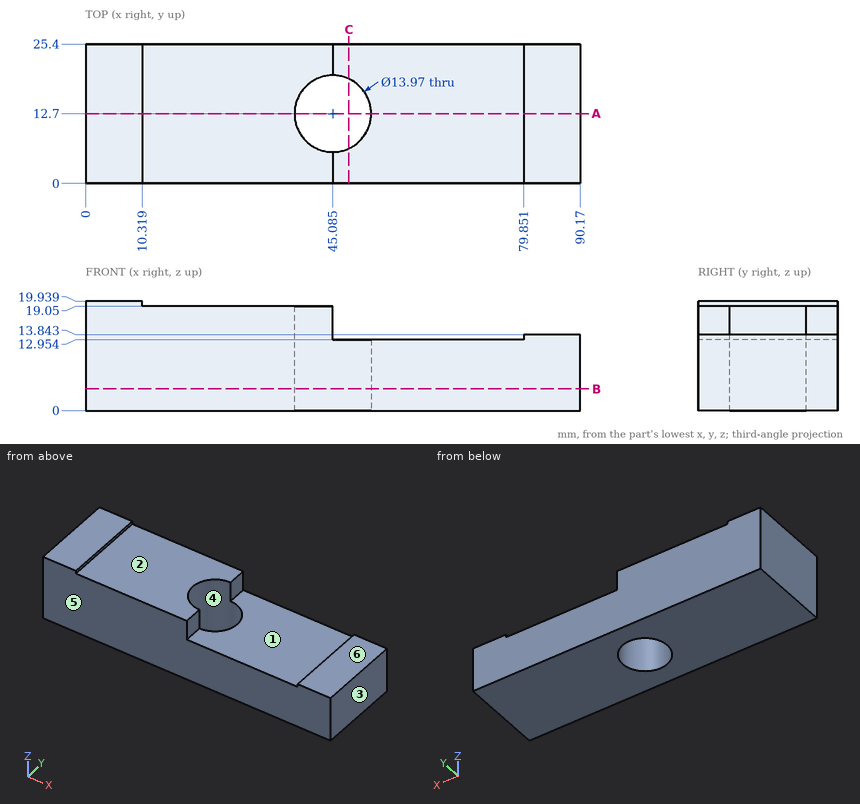
The drawing under review shows one solid part. Ordinate dimensions are in mm from its lowest x, y, z. A direction names the side the tool comes from. Round coordinates to 2 decimals unless told otherwise and drop trailing zeros. Order: outer loops, then holes, each group sorted by start corner. A loop starts at its lowest first (then second) coordinate and runs counter-clockwise, first axis right, second up. Notation, with made-up numbers: (-12, 0.25) -> (-7, 0.25) arc R26 cw to (-7, 24.25) -> close; hole circle Ø1 at (42, 81.25). An arc over 180 degrees is marked (long way). Use a Markdown table: item, result.
Item 1: Take a section at C-C (x = 48). State the section outline as (y, z) points, plus the area to 3 significant figures.
Resolved:
| item | result |
|---|---|
| outline | (0, 0) -> (6.35, 0) -> (6.35, 12.95) -> (0, 12.95) -> close; (19.05, 0) -> (25.4, 0) -> (25.4, 12.95) -> (19.05, 12.95) -> close |
| area | 165 mm² |
Item 2: Machinability: for the marked faces 1, 2 and 3, which of the approach directions +Z, -Z, +X, -X, +Y, -Y give a long, thin tool a straight path to every point of the face, cutting with its end or side? Answer none if there is none.
Resolved:
| item | result |
|---|---|
| face 1 | +Z, +Y, -Y |
| face 2 | +Z, +X, +Y, -Y |
| face 3 | +Z, -Z, +X, +Y, -Y |
Item 3: For line 1 along X through (y, z) = (12.7, 4); line 2 along Y through (x, z) = (45.5, 2.5); line 3 along Z through (x, y) = (53.5, 2.75), list the stretches that pass through material, from the lowest coordinate up. Write a range as [from, to].
Resolved:
| item | result |
|---|---|
| line 1 | x = [0, 38.1], [52.07, 90.17] |
| line 2 | y = [0, 5.73], [19.67, 25.4] |
| line 3 | z = [0, 12.95] |
Item 4: For pin 1 (6 mm diameter, centred on x = 37, y = 12.5, fed in from +Z); pin 2 (0.7 mm diameter, centred on y = 16.5, z = 19.5, fed in from +X); pin 3 (5 mm diameter, centred on x = 84, y = 13, fed in from +Z), all flat-tipped, find the tip position at first contact; note any pin that passes through.
Resolved:
| item | result |
|---|---|
| pin 1 | stops at z = 19.05 |
| pin 2 | stops at x = 10.32 |
| pin 3 | stops at z = 13.84 |
Item 5: Draft analysis for pull direction Y (two halves, no side actions). For the marked faces 4, 5 and 6, state which applies: +Y half, -Y half, draft (parallel to the pull), parting line (faces both ways), or undercut.
Resolved:
| item | result |
|---|---|
| face 4 | undercut |
| face 5 | -Y half |
| face 6 | draft |
Item 6: Take a section at A-A (y = 12.7). State the section outline as (x, z) points.
Resolved:
| item | result |
|---|---|
| outline | (0, 0) -> (38.1, 0) -> (38.1, 19.05) -> (10.32, 19.05) -> (10.32, 19.94) -> (0, 19.94) -> close; (52.07, 0) -> (90.17, 0) -> (90.17, 13.84) -> (79.85, 13.84) -> (79.85, 12.95) -> (52.07, 12.95) -> close |
Item 7: Take a section at B-B (z = 4). State the section outline as (x, y) points (1 decimal).
Resolved:
| item | result |
|---|---|
| outline | (0, 0) -> (90.2, 0) -> (90.2, 25.4) -> (0, 25.4) -> close; hole circle Ø14 at (45.1, 12.7) |
